from build123d import *

# Parameters (mm, degrees)
SKETCH1_W           = 292.1
SKETCH1_H           = 89.8
SKETCH1_R           = 14.2875
SKETCH1_R_2         = 2.54
SKETCH1_R_3         = 17.145
BOSS_EXTRUDE1_DEPTH = 6.35
SKETCH2_R           = 2.05
CUT_EXTRUDE1_DEPTH  = 10
SKETCH3_R           = 1.55
SKETCH3_R_2         = 2.05
SKETCH3_R_3         = 1.5
CUT_EXTRUDE2_DEPTH  = 10
FILLET1_R           = 2
SKETCH4_R           = 2.05
SKETCH4_R_2         = 1.778
CUT_EXTRUDE4_DEPTH  = 7.35


with BuildPart() as part:
    # Sketch1 → Boss-Extrude1 (new body)
    with BuildSketch(Plane.XY):
        with Locations((146.05, 44.9)):
            Rectangle(SKETCH1_W, SKETCH1_H)
        with Locations((146.05, 44.9)):
            Circle(SKETCH1_R, mode=Mode.SUBTRACT)
        with Locations((103.051585406, 62.859439014)):
            Circle(SKETCH1_R_2, mode=Mode.SUBTRACT)
        with Locations((103.049439014, 26.938414594)):
            Circle(SKETCH1_R_2, mode=Mode.SUBTRACT)
        with Locations((67.128414594, 26.940560986)):
            Circle(SKETCH1_R_2, mode=Mode.SUBTRACT)
        with Locations((67.130560986, 62.861585406)):
            Circle(SKETCH1_R_2, mode=Mode.SUBTRACT)
        with Locations((85.09, 44.9)):
            Circle(SKETCH1_R_3, mode=Mode.SUBTRACT)
        with Locations((189.050560986, 62.861585406)):
            Circle(SKETCH1_R_2, mode=Mode.SUBTRACT)
        with Locations((224.971585406, 62.859439014)):
            Circle(SKETCH1_R_2, mode=Mode.SUBTRACT)
        with Locations((224.969439014, 26.938414594)):
            Circle(SKETCH1_R_2, mode=Mode.SUBTRACT)
        with Locations((189.048414594, 26.940560986)):
            Circle(SKETCH1_R_2, mode=Mode.SUBTRACT)
        with Locations((207.01, 44.9)):
            Circle(SKETCH1_R_3, mode=Mode.SUBTRACT)
    extrude(amount=BOSS_EXTRUDE1_DEPTH)

    # Sketch2 → Cut-Extrude1 (cut)
    with BuildSketch(Plane.XY.offset(6.35)):
        with Locations((118.55, 20)):
            Circle(SKETCH2_R)
        with Locations((118.55, 69.8)):
            Circle(SKETCH2_R)
        with Locations((173.55, 20)):
            Circle(SKETCH2_R)
        with Locations((173.55, 69.8)):
            Circle(SKETCH2_R)
    extrude(amount=-CUT_EXTRUDE1_DEPTH, mode=Mode.SUBTRACT)

    # Sketch3 → Cut-Extrude2 (cut)
    with BuildSketch(Plane.XY.offset(6.35)):
        with Locations((284.6, 7.5)):
            Circle(SKETCH3_R)
        with Locations((7.5, 7.5)):
            Circle(SKETCH3_R)
        with Locations((7.5, 82.3)):
            Circle(SKETCH3_R)
        with Locations((284.6, 82.3)):
            Circle(SKETCH3_R)
        with Locations((274.6, 20)):
            Circle(SKETCH3_R_2)
        with Locations((17.5, 20)):
            Circle(SKETCH3_R_2)
        with Locations((17.5, 69.8)):
            Circle(SKETCH3_R_2)
        with Locations((274.6, 69.8)):
            Circle(SKETCH3_R_2)
        with Locations((173.55, 7.5)):
            Circle(SKETCH3_R_3)
        with Locations((173.55, 82.3)):
            Circle(SKETCH3_R_3)
        with Locations((118.55, 82.3)):
            Circle(SKETCH3_R_3)
        with Locations((118.55, 7.5)):
            Circle(SKETCH3_R_3)
    extrude(amount=-CUT_EXTRUDE2_DEPTH, mode=Mode.SUBTRACT)

    # Fillet1
    fillet1_edges = [part.edges().sort_by_distance(p)[0] for p in [
        (0, 89.8, 3.175),
        (292.1, 89.8, 3.175),
        (292.1, 0, 3.175),
        (0, 0, 3.175),
    ]]
    fillet(fillet1_edges, radius=FILLET1_R)

    # Sketch4 → Cut-Extrude4 (cut, through all)
    with BuildSketch(Plane.XY.offset(6.35)):
        with Locations((233.55, 20)):
            Circle(SKETCH4_R)
        with Locations((233.55, 69.8)):
            Circle(SKETCH4_R_2)
        with Locations((58.55, 69.8)):
            Circle(SKETCH4_R_2)
        with Locations((58.55, 20)):
            Circle(SKETCH4_R_2)
    extrude(amount=-CUT_EXTRUDE4_DEPTH, mode=Mode.SUBTRACT)


solid = part.part
Design review of the part built by this model. Coordinates are the model's own, in mm. Coordinates: 2 decimals unless noted, no trailing zeros. Loops run counter-clockwise (first coordinate to the right, second up) from the corner with the lowest first, then second, coordinate; pieces in that order, holes last. Notation, with made-up numbers: M 17.5,26.25 L 29.5,26.25 A8 ccw 29.5,40.25 Z; hole C 42,0 d2. An arc over 180 degrees is marked long. Answer as CSV lines item,"result".
Item 1: Add section B-B on y = 41. State the section outline as (x, z) points, plus the area to 3 significant figures.
Answer list:
outline,"M 0,0 L 68.39,0 L 68.39,6.35 L 0,6.35 Z; M 101.79,0 L 132.31,0 L 132.31,6.35 L 101.79,6.35 Z; M 159.79,0 L 190.31,0 L 190.31,6.35 L 159.79,6.35 Z; M 223.71,0 L 292.1,0 L 292.1,6.35 L 223.71,6.35 Z"
area,"1,260 mm²"
Item 2: Add section D-D on z = 3. Count the separate pieces of the cut face and the enclosed holes in it, plus the area to 3 significant figures.
Answer list:
separate pieces,"1"
enclosed holes,"31"
area,"23,400 mm²"
Item 3: For probe 1 along Y at (x, z) = (58.55, 2.5); probe 2 along Y at (x, z) = (118.55, 4.75); probe 3 along Y at (x, z) = (284.6, 4), list the stretches that pass through material, from the lowest coordinate up.
Answer list:
probe 1,"0 to 18.22, 21.78 to 68.02, 71.58 to 89.8"
probe 2,"0 to 6, 9 to 17.95, 22.05 to 67.75, 71.85 to 80.8, 83.8 to 89.8"
probe 3,"0 to 5.95, 9.05 to 80.75, 83.85 to 89.8"
Item 4: Add section A-A on x = 146.05. State the section outline as (y, z) points, plus the area to 3 significant figures.
Answer list:
outline,"M 0,0 L 30.61,0 L 30.61,6.35 L 0,6.35 Z; M 59.19,0 L 89.8,0 L 89.8,6.35 L 59.19,6.35 Z"
area,"389 mm²"
Item 5: The part is to be moulded in two halves that separate along X. For faces 1 (the face through (105.474, 63.622, 3.131)), 2 (the face through (292.1, 44, 3)), 3 (the face through (0, 44, 3)), 4 (the face through (144, 89.8, 3)), say which applies: pulls with the +X half, pulls with the -X half, needs draft (parallel to the pull), parting line crosses it, or undercut.
Answer list:
face 1,"undercut"
face 2,"pulls with the +X half"
face 3,"pulls with the -X half"
face 4,"needs draft"
Item 6: Add section C-C on x = 85.09. State the section outline as (y, z) points (3 decimals), plus the area to 3 significant figures.
Answer list:
outline,"M 0,0 L 27.755,0 L 27.755,6.35 L 0,6.35 Z; M 62.045,0 L 89.8,0 L 89.8,6.35 L 62.045,6.35 Z"
area,"352 mm²"
